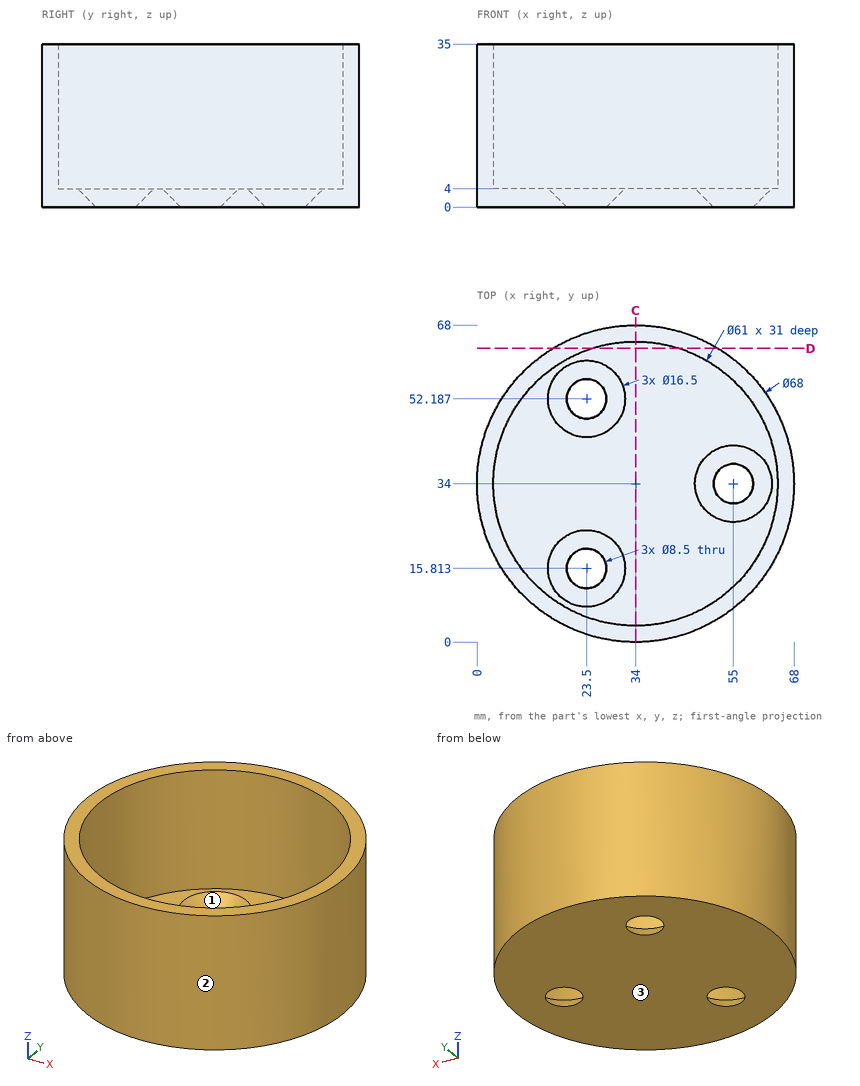
Geometry check sheet. Reference: drawing and pictorial views, mm from the part's lowest x, y, z. Give positions to 0.01 mm unless a question says otherwise; leave off trailing zeros. Order: outer loops, then holes, each group sorted by start corner. A loop starts at its lowest first (then second) coordinate and runs counter-clockwise, first axis right, second up. Notation, with made-up numbers: (4, 43.25) - (44, 43.25) arc R13 cw to (44, 66.25) - close; hole circle Ø8 at (59, 84.5). An arc over 180 degrees is marked (long way). Use one line per item in the form item = value.
1) Draft check along Y on the marked faces 1, 2 and 3. Enter one of: released by +Y, released by -Y, zero draft, split by the parting line, or undercut.
Working result:
face_1 = undercut
face_2 = split by the parting line
face_3 = zero draft
2) Depth check by flat-ended pin: pin 1 Ø8 at (x, z) = (42.5, 31) entering from +Y; pin 2 Ø12 at (y, z) = (26.5, 11) entering from -X; pin 3 Ø3 at (y, z) = (18.5, 21.5) entering from +X. Enter the tip coordinate at first touch or a pass-through.
Working result:
pin_1 = 67.7
pin_2 = 0.03
pin_3 = 64.98
3) Sectioned sample at D-D (y = 63). Record the boundary of the cut face in (x, z).
Working result:
outline = (16.25, 0) - (51.75, 0) - (51.75, 35) - (43.45, 35) - (43.45, 4) - (24.55, 4) - (24.55, 35) - (16.25, 35) - close
4) Material ranges on probe 1 along Y at (x, z) = (23.5, 0.05) (1 decimal); probe 2 along Z at (x, y) = (50.5, 48); probe 3 along X at (y, z) = (34, 26), recorded low to high. Write a range as from..to.
Working result:
probe_1 = 1.7..11.5, 20.1..47.9, 56.5..66.3
probe_2 = 0..4
probe_3 = 0..3.5, 64.5..68
5) Sectioned sample at C-C (x = 34). Record the boundary of the cut face in (y, z).
Working result:
outline = (0, 0) - (68, 0) - (68, 35) - (64.5, 35) - (64.5, 4) - (3.5, 4) - (3.5, 35) - (0, 35) - close
